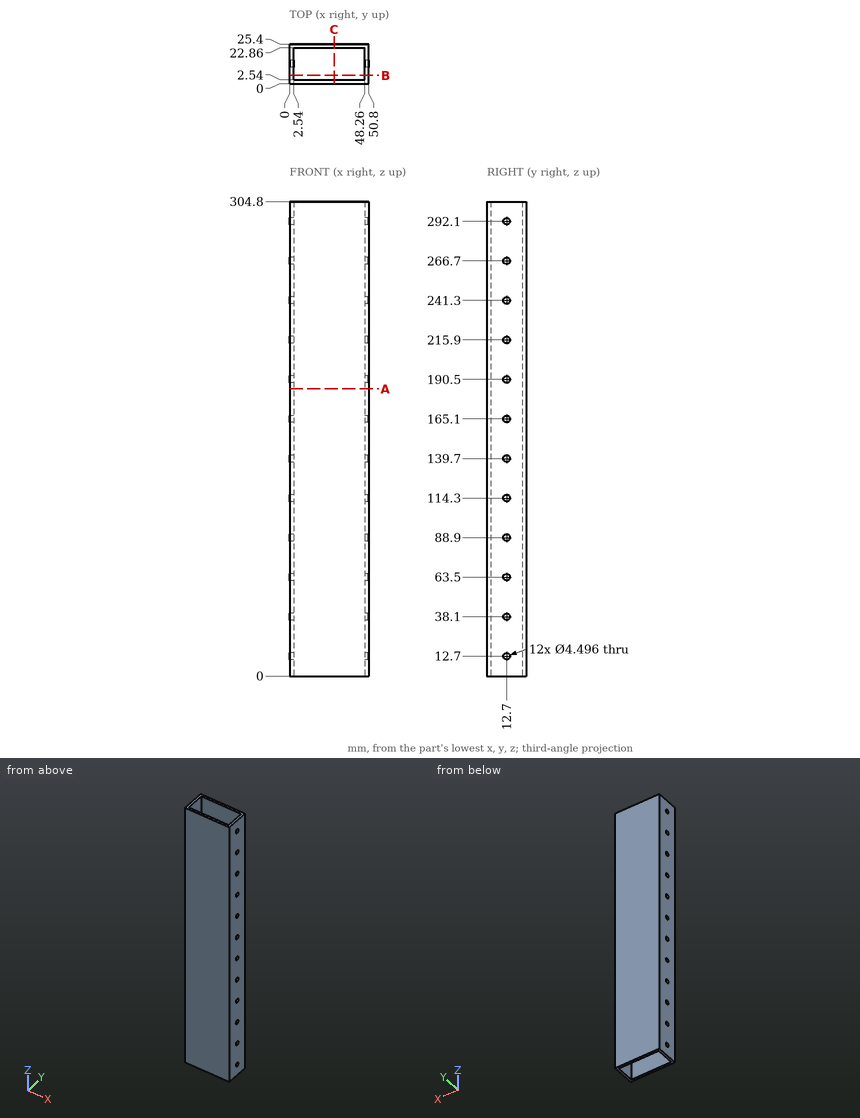
Could you check a few things on this drawing? It's one solid part, dimensions in mm from its lowest x, y, z. Coordinates: 2 decimals unless noted, no trailing zeros. Order: outer loops, then holes, each group sorted by start corner. A loop starts at its lowest first (then second) coordinate and runs counter-clockwise, first axis right, second up. Notation, with made-up numbers: M 86.25,64 L 123.25,64 A10 ccw 123.25,73 Z; hole C 36,15.5 d9. An arc over 180 degrees is marked long. Answer as a JSON object with one key per item and string values. Group by question number.
(1) I need wall thicknesses on probe 1 along X at (y, z) = (4.5, 32); probe 2 along Y at (x, z) = (50.1, 139.7); probe 3 along Y at (x, z) = (16, 250.5). Which ranges of each line are inside material? Lowest first, please.
(2) Suppose I cut it at A-A, the plane z = 184.5. Please give me the cut outline in (x, y), then the cut area to 3 significant figures.
(3) Suppose I cut it at C-C, the plane x = 28.5. Please give me the cut outline in (y, z).
(4) Suppose I cut it at B-B, the plane y = 5.25. Please give me the cut outline in (x, z).
(5) For pin 1 (4 mm diameter, centred on y = 12.7, z = 241.3, fed in from -X); pin 2 (7 mm diameter, centred on y = 12.7, z = 292.1, fed in from -X), each with a flat end and sliding along its axis, tell me the tip position at first contact or that it passes through.
Values found:
{
 "1": {"probe 1": "x = 0 to 2.54, 48.26 to 50.8", "probe 2": "y = 0 to 10.45, 14.95 to 25.4", "probe 3": "y = 0 to 2.54, 22.86 to 25.4"},
 "2": {"outline": "M 0,0 L 50.8,0 L 50.8,25.4 L 0,25.4 Z; hole M 2.54,2.54 L 48.26,2.54 L 48.26,22.86 L 2.54,22.86 Z", "area": "361 mm^2"},
 "3": {"outline": "M 0,0 L 2.54,0 L 2.54,304.8 L 0,304.8 Z; M 22.86,0 L 25.4,0 L 25.4,304.8 L 22.86,304.8 Z"},
 "4": {"outline": "M 0,0 L 2.54,0 L 2.54,304.8 L 0,304.8 Z; M 48.26,0 L 50.8,0 L 50.8,304.8 L 48.26,304.8 Z"},
 "5": {"pin 1": "passes through", "pin 2": "stops at x = 0"}
}
